```python
from build123d import *

# Parameters (mm, degrees)
SKETCH1_W           = 68
SKETCH1_H           = 33
BOSS_EXTRUDE1_DEPTH = 20
SKETCH2_R           = 1.625
BOSS_EXTRUDE2_DEPTH = 1.175
FILLET1_R           = 1
CUT_EXTRUDE1_DEPTH  = 13
SKETCH5_W           = 4.75
SKETCH5_H           = 20
BOSS_EXTRUDE3_DEPTH = 17
SKETCH7_R           = 2.25
CUT_EXTRUDE2_DEPTH  = 60.216810324
CUT_EXTRUDE3_DEPTH  = 3.2
FILLET2_R           = 10
FILLET4_R           = 3
FILLET5_R           = 1


with BuildPart() as part:
    # Sketch1 → Boss-Extrude1 (new body)
    with BuildSketch(Plane.XY):
        Rectangle(SKETCH1_W, SKETCH1_H)
        Polygon((-27, 14.5), (-32, 9.5), (-32, -9.5), (-27, -14.5), (27, -14.5), (32, -9.5), (32, 9.5), (27, 14.5), align=None, mode=Mode.SUBTRACT)
    extrude(amount=BOSS_EXTRUDE1_DEPTH)

    # Sketch2 → Boss-Extrude2 (add)
    with BuildSketch(Plane.XY.offset(20)):
        with Locations((31.75, -14.25)):
            Circle(SKETCH2_R)
        with Locations(Location((31.75, 14.25, 0), (0, 0, 180))):
            Circle(SKETCH2_R)
        with Locations((-31.75, 14.25)):
            Circle(SKETCH2_R)
        with Locations(Location((-31.75, -14.25, 0), (0, 0, 180))):
            Circle(SKETCH2_R)
    extrude(amount=BOSS_EXTRUDE2_DEPTH)

    # Fillet1
    fillet1_edges = [part.edges().sort_by_distance(p)[0] for p in [
        (34, -16.5, 10),
        (-34, -16.5, 10),
        (-34, 16.5, 10),
        (34, 16.5, 10),
    ]]
    fillet(fillet1_edges, radius=FILLET1_R)

    # Sketch3 → Cut-Extrude1 (cut)
    with BuildSketch(Plane.ZY.offset(34)):
        with BuildLine():
            Line((7, -1.75), (-7, -1.75))
            ThreePointArc((-7, -1.75), (-8.75, 0), (-7, 1.75))
            Line((-7, 1.75), (7, 1.75))
            ThreePointArc((7, 1.75), (8.75, 0), (7, -1.75))
        make_face()
    extrude(amount=-CUT_EXTRUDE1_DEPTH, mode=Mode.SUBTRACT)

    # Sketch5 → Boss-Extrude3 (add)
    with BuildSketch(Plane.XZ.offset(16.5)):
        with Locations((7.625, 10)):
            Rectangle(SKETCH5_W, SKETCH5_H)
        with Locations((-7.625, 10)):
            Rectangle(SKETCH5_W, SKETCH5_H)
    extrude(amount=BOSS_EXTRUDE3_DEPTH)

    # Sketch7 → Cut-Extrude2 (cut, through all)
    with BuildSketch(Plane.ZY.offset(10)):
        with Locations((10, -24.5)):
            Circle(SKETCH7_R)
    extrude(amount=-CUT_EXTRUDE2_DEPTH, mode=Mode.SUBTRACT)

    # Sketch8 → Cut-Extrude3 (cut)
    with BuildSketch(Plane.ZY.offset(10)):
        Polygon((5.554402927, -24.5), (7.777201464, -28.35), (12.222798536, -28.35), (14.445597073, -24.5), (12.222798536, -20.65), (7.777201464, -20.65), align=None)
    extrude(amount=-CUT_EXTRUDE3_DEPTH, mode=Mode.SUBTRACT)

    # Fillet2
    fillet2_edges = [part.edges().sort_by_distance(p)[0] for p in [
        (7.625, -33.5, 0),
        (7.625, -33.5, 20),
        (-7.625, -33.5, 0),
        (-7.625, -33.5, 20),
    ]]
    fillet(fillet2_edges, radius=FILLET2_R - 0.0001)  # a hair under: the kernel refuses the full size

    # Fillet4
    fillet4_edges = [part.edges().sort_by_distance(p)[0] for p in [
        (10, -16.5, 10),
        (-10, -16.5, 10),
    ]]
    fillet(fillet4_edges, radius=FILLET4_R)

    # Fillet5
    fillet5_edges = [part.edges().sort_by_distance(p)[0] for p in [
        (5.25, -16.5, 10),
        (-5.25, -16.5, 10),
    ]]
    fillet(fillet5_edges, radius=FILLET5_R)


solid = part.part
```
CAD build for the part. Positions are in the model's coordinates, mm. A direction names the side the tool comes from. Give positions to 0.01 mm unless a question says otherwise; leave off trailing zeros. Order: outer loops, then holes, each group sorted by start corner. A loop starts at its lowest first (then second) coordinate and runs counter-clockwise, first axis right, second up. Notation, with made-up numbers: M 45,34.5 L 95,34.5 A9 ccw 95,51.5 Z; hole C 26.25,30.25 d8. An arc over 180 degrees is marked long. Put each result on its own line as item: value. Start each with the question number.
(1) Saw through at B-B, the plane x = -8.5. Give the number of separate pieces and of enclosed holes in the cut face, then the cut area to 3 significant figures.
(2) Saw through at C-C, the plane x = 23.5. Write the cut outline in (y, z), then the cut area to 3 significant figures.
(3) Drill centre lines: line 1 along Y through (x, z) = (-6.25, 10); line 2 along X through (y, z) = (3.5, 2.25); line 3 along Y through (x, z) = (-27, 8). Where is each one in solid material? Low to high.
(4) Which spindle directions (+Z, -Z, +X, -X, +Y, -Y) get a long thin tool onto all of the face, cutting with end or side? Do faces 4 (the flat face through (10, -26, 12)), 5 (the flat face through (-32, 0, 10)), 6 (the cylindrical face through (33.04, 15.24, 20.58)), 7 (the flat face through (-23, -16.5, 10)). Say none if no direction does.
(5) Saw through at D-D, the plane z = 16.5. Write the cut outline in (x, y).
(6) Flat gauge pins, fed straight in: pin 1 Ø5 at (y, z) = (-22.5, 6.5) entering from +X; pin 2 Ø6 at (y, z) = (-24.5, 11.5) entering from -X; pin 3 Ø8 at (x, z) = (-21.5, 16.5) entering from -Y; pin 4 Ø3.5 at (y, z) = (-24.5, 10) entering from -X. Where does each tip first touch, or does it go through?
(7) Mould opens along Z. For faces 1 (the flat face through (-8.42, -26.45, 13.32)), 2 (the cylindrical face through (30.46, -15.24, 20.58)), 3 (the flat face through (0, -15, 20)) say: +Z half, -Z half, draft (parallel to the pull), parting line (faces both ways), or undercut.
(8) Saw through at A-A, the plane y = 0. Write the cut outline in (x, z), then the cut area to 3 significant figures.
Check result:
1. separate pieces: 2
1. enclosed holes: 1
1. area: 326 mm2
2. outline: M -16.5,0 L -14.5,0 L -14.5,20 L -16.5,20 Z; M 14.5,0 L 16.5,0 L 16.5,20 L 14.5,20 Z
2. area: 80.0 mm2
3. line 1: y = -33.5 to -26.75, -22.25 to -14.5, 14.5 to 16.5
3. line 2: x = -34 to -32, 32 to 34
3. line 3: y = -16.5 to -14.5, 14.5 to 16.5
4. face 4: +Z, -Z, +X, -Y
4. face 5: +Z, -Z
4. face 6: +Z
4. face 7: +Z, -Z, -X, -Y
5. outline: M -34,-15.5 A1 ccw -33,-16.5 L -13,-16.5 A3 cw -10,-19.5 L -10,-31.1 L -5.25,-31.1 L -5.25,-17.5 A1 cw -4.25,-16.5 L 4.25,-16.5 A1 cw 5.25,-17.5 L 5.25,-31.1 L 10,-31.1 L 10,-19.5 A3 cw 13,-16.5 L 33,-16.5 A1 ccw 34,-15.5 L 34,15.5 A1 ccw 33,16.5 L -33,16.5 A1 ccw -34,15.5 Z; hole M -32,-9.5 L -27,-14.5 L 27,-14.5 L 32,-9.5 L 32,9.5 L 27,14.5 L -27,14.5 L -32,9.5 Z
6. pin 1: stops at x = 10
6. pin 2: stops at x = -10
6. pin 3: stops at y = -16.5
6. pin 4: passes through
7. face 1: undercut
7. face 2: draft
7. face 3: +Z half
8. outline: M -34,8.75 L -32,8.75 L -32,20 L -34,20 Z; M 32,0 L 34,0 L 34,20 L 32,20 Z
8. area: 62.5 mm2
